Read the model definition and answer for the solid it produces. Units are mm, in the model's axes. Face numbers are marked on the shaded views. A direction names the side the tool comes from. Give positions to 0.01 mm unless a question says otherwise; leave off trailing zeros. Write each loop counter-clockwise with the first axis right and the second up, starting at its lowest first coordinate (ties: lowest second). Pieces come first, ordered by that corner, then holes. Notation, with made-up numbers: M 53.25,76 L 107.25,76 A15 cw 107.25,99 Z; hole C 83,86.25 d2. An arc over 180 degrees is marked long. Put each result on its own line as item: value.
from build123d import *

# Parameters (mm, degrees)
F0_W      = 27.6
F0_H      = 27.6
F1_DEPTH  = 30
F2_R      = 2.5
F3_R      = 10.975
F4_DEPTH  = 14
F5_R      = 8.5
F6_DEPTH  = 3
F7_R      = 10.5
F7_R_2    = 8.5
F8_DEPTH  = 5
F9_W      = 29
F9_H      = 29
F10_DEPTH = 5
F11_R     = 2
F12_W     = 32.5
F12_H     = 32.5
F13_DEPTH = 5
F14_R     = 2
F15_W     = 30
F15_H     = 30
F16_DEPTH = 8
F17_SIZE  = 3
F18_R     = 8.88
F19_DEPTH = 15
F20_R     = 5.075
F21_DEPTH = 140


with BuildPart() as f1:
    # F0 (on Top) → F1 (new body)
    with BuildSketch(Plane.XY):
        Rectangle(F0_W, F0_H)
    extrude(amount=F1_DEPTH)

    # F2
    f2_edges = [f1.edges().sort_by_distance(p)[0] for p in [
        (-13.8, -13.8, 15),
        (13.8, -13.8, 15),
        (13.8, 13.8, 15),
        (-13.8, 13.8, 15),
    ]]
    fillet(f2_edges, radius=F2_R)

    # F3 (on face) → F4 (join)
    with BuildSketch(Plane.XZ.offset(13.8)):
        with Locations((0, 19)):
            Circle(F3_R)
    extrude(amount=F4_DEPTH)

    # F5 (on face) → F6 (join)
    with BuildSketch(Plane.XZ.offset(27.8)):
        with Locations((0, 19)):
            Circle(F5_R)
    extrude(amount=F6_DEPTH)

    # F7 (on face) → F8 (join)
    with BuildSketch(Plane.XZ.offset(30.8)):
        with Locations((0, 19)):
            Circle(F7_R)
        with Locations((0, 19)):
            Circle(F7_R_2, mode=Mode.SUBTRACT)
        with Locations((0, 19)):
            Circle(F7_R_2)
    extrude(amount=F8_DEPTH)

    # F9 (on face) → F10 (join)
    with BuildSketch(Plane(origin=(0, 0, 0), x_dir=(1, 0, 0), z_dir=(0, 0, -1))):
        Rectangle(F9_W, F9_H)
        with BuildLine():
            Line((-11.3, 13.8), (11.3, 13.8))
            ThreePointArc((11.3, 13.8), (13.067766953, 13.067766953), (13.8, 11.3))
            Line((13.8, 11.3), (13.8, -11.3))
            ThreePointArc((13.8, -11.3), (13.067766953, -13.067766953), (11.3, -13.8))
            Line((11.3, -13.8), (-11.3, -13.8))
            ThreePointArc((-11.3, -13.8), (-13.067766953, -13.067766953), (-13.8, -11.3))
            Line((-13.8, -11.3), (-13.8, 11.3))
            ThreePointArc((-13.8, 11.3), (-13.067766953, 13.067766953), (-11.3, 13.8))
        make_face(mode=Mode.SUBTRACT)
        with BuildLine():
            ThreePointArc((13.8, 11.3), (13.067766953, 13.067766953), (11.3, 13.8))
            Line((11.3, 13.8), (-11.3, 13.8))
            ThreePointArc((-11.3, 13.8), (-13.067766953, 13.067766953), (-13.8, 11.3))
            Line((-13.8, 11.3), (-13.8, -11.3))
            ThreePointArc((-13.8, -11.3), (-13.067766953, -13.067766953), (-11.3, -13.8))
            Line((-11.3, -13.8), (11.3, -13.8))
            ThreePointArc((11.3, -13.8), (13.067766953, -13.067766953), (13.8, -11.3))
            Line((13.8, -11.3), (13.8, 11.3))
        make_face()
    extrude(amount=F10_DEPTH)

    # F11
    f11_edges = [f1.edges().sort_by_distance(p)[0] for p in [
        (-14.5, 14.5, -2.5),
        (-14.5, -14.5, -2.5),
        (14.5, -14.5, -2.5),
        (14.5, 14.5, -2.5),
    ]]
    fillet(f11_edges, radius=F11_R)

    # F12 (on face) → F13 (join)
    with BuildSketch(Plane(origin=(0, 0, -5), x_dir=(1, 0, 0), z_dir=(0, 0, -1))):
        Rectangle(F12_W, F12_H)
        with BuildLine():
            Line((12.5, -14.5), (-12.5, -14.5))
            ThreePointArc((-12.5, -14.5), (-13.9142135624, -13.9142135624), (-14.5, -12.5))
            Line((-14.5, -12.5), (-14.5, 12.5))
            ThreePointArc((-14.5, 12.5), (-13.9142135624, 13.9142135624), (-12.5, 14.5))
            Line((-12.5, 14.5), (12.5, 14.5))
            ThreePointArc((12.5, 14.5), (13.9142135624, 13.9142135624), (14.5, 12.5))
            Line((14.5, 12.5), (14.5, -12.5))
            ThreePointArc((14.5, -12.5), (13.9142135624, -13.9142135624), (12.5, -14.5))
        make_face(mode=Mode.SUBTRACT)
        with BuildLine():
            ThreePointArc((-14.5, -12.5), (-13.9142135624, -13.9142135624), (-12.5, -14.5))
            Line((-12.5, -14.5), (12.5, -14.5))
            ThreePointArc((12.5, -14.5), (13.9142135624, -13.9142135624), (14.5, -12.5))
            Line((14.5, -12.5), (14.5, 12.5))
            ThreePointArc((14.5, 12.5), (13.9142135624, 13.9142135624), (12.5, 14.5))
            Line((12.5, 14.5), (-12.5, 14.5))
            ThreePointArc((-12.5, 14.5), (-13.9142135624, 13.9142135624), (-14.5, 12.5))
            Line((-14.5, 12.5), (-14.5, -12.5))
        make_face()
    extrude(amount=F13_DEPTH)

    # F14
    f14_edges = [f1.edges().sort_by_distance(p)[0] for p in [
        (16.25, -16.25, -7.5),
        (16.25, 16.25, -7.5),
        (-16.25, 16.25, -7.5),
        (-16.25, -16.25, -7.5),
    ]]
    fillet(f14_edges, radius=F14_R)

    # F15 (on face) → F16 (join)
    with BuildSketch(Plane(origin=(0, 0, -10), x_dir=(1, 0, 0), z_dir=(0, 0, -1))):
        Rectangle(F15_W, F15_H)
    extrude(amount=F16_DEPTH)

    # F17
    f17_edges = [f1.edges().sort_by_distance(p)[0] for p in [
        (-15, -15, -14),
        (15, -15, -14),
        (15, 15, -14),
        (-15, 15, -14),
    ]]
    chamfer(f17_edges, length=F17_SIZE)

    # F18 (on face) → F19 (join)
    with BuildSketch(Plane(origin=(0, 0, -18), x_dir=(1, 0, 0), z_dir=(0, 0, -1))):
        Circle(F18_R)
    extrude(amount=F19_DEPTH)

    # F20 (on face) → F21 (join)
    with BuildSketch(Plane(origin=(0, 0, -33), x_dir=(1, 0, 0), z_dir=(0, 0, -1))):
        Circle(F20_R)
    extrude(amount=F21_DEPTH)


solid = f1.part
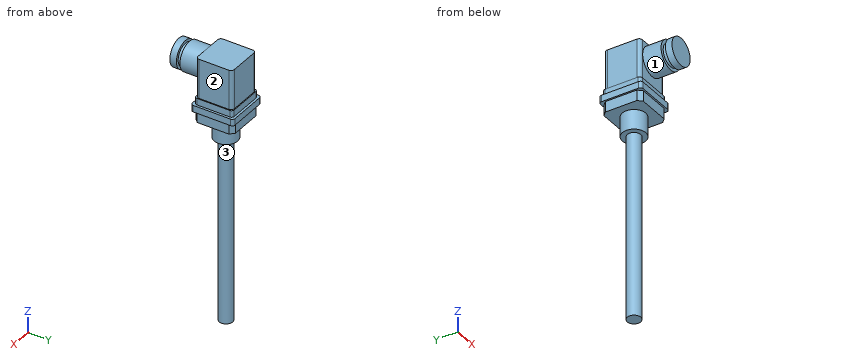
(1) Section D-D on z = -130 is taken. Determine the outline of the cut face in (x, y) (3 decimals).
Result:
outline: C 0,0 d10.15
(2) Section C-C on y = -19.5 is taken. Determine the outline of the cut face in (x, z) (3 decimals).
Result:
outline: C 0,19 d21.95
(3) Section A-A on y = 0 is taken. Determine the outline of the cut face in (x, z) (3 decimals).
Result:
outline: M -16.25,-10 L -15,-10 L -15,-18 L -8.88,-18 L -8.88,-33 L -5.075,-33 L -5.075,-173 L 5.075,-173 L 5.075,-33 L 8.88,-33 L 8.88,-18 L 15,-18 L 15,-10 L 16.25,-10 L 16.25,-5 L 14.5,-5 L 14.5,0 L 13.8,0 L 13.8,30 L -13.8,30 L -13.8,0 L -14.5,0 L -14.5,-5 L -16.25,-5 Z
(4) Which of the six approach directions +Z, -Z, +X, -X, +Y, -Y give full straight-line access (tool end or side, diameter ignored) to the marked faces 1, 2 and 3?
Result:
face 1: -Y
face 2: +Z, +X, +Y, -Y
face 3: -Z
(5) Section B-B on z = 19 is taken. Determine the outline of the cut face in (x, y) (3 decimals), and give its area (3 significant figures).
Result:
outline: M -13.8,-11.3 A2.5 ccw -11.3,-13.8 L -10.975,-13.8 L -10.975,-27.8 L -8.5,-27.8 L -8.5,-30.8 L -10.5,-30.8 L -10.5,-35.8 L 10.5,-35.8 L 10.5,-30.8 L 8.5,-30.8 L 8.5,-27.8 L 10.975,-27.8 L 10.975,-13.8 L 11.3,-13.8 A2.5 ccw 13.8,-11.3 L 13.8,11.3 A2.5 ccw 11.3,13.8 L -11.3,13.8 A2.5 ccw -13.8,11.3 Z
area: 1,220 mm²
(6) Given pin 1 Ø4 at (x, y) = (11, -20.5) entering from +Z; pin 2 Ø2 at (x, z) = (2, -47) entering from +Y; pin 3 Ø4 at (x, z) = (-2, -13.5) entering from +Y, each flat-ended and moving along its own axis, determine where each tip first touches the part or whether it passes through.
Result:
pin 1: stops at z = 25.28
pin 2: stops at y = 4.98
pin 3: stops at y = 15
(7) Straight lines are drawn through the part: line 1 along Y through (x, z) = (8, 14.5); line 2 along Z through (x, y) = (-8, 11.5); line 3 along Z through (x, y) = (-4.5, 5). For each, find the intervals that lie inside material, in ascending order. Write a range as from..to.
Result:
line 1: y = -35.8..-30.8, -27.8..13.8
line 2: z = -18..30
line 3: z = -33..30
